Could you check a few things on this model? Use its own coordinates, in mm. A direction names the side the tool comes from. Give positions to 0.01 mm unless a question says otherwise; leave off trailing zeros. Loops run counter-clockwise (first coordinate to the right, second up) from the corner with the lowest first, then second, coordinate; pieces in that order, holes last.
1. For P1, Ø6, axis at x = 77.5, y = 2.5, coming from the -Z side; P2, Ø6.5, axis at x = 66.94, z = 2.99, coming from the +Y side; P3, Ø1, axis at x = -1.5, y = 5, coming from the -Z side, each with a flat end and sliding along its axis, tell me the tip position at first contact or that it passes through.
2. Imagine slicing it at C-C (x = -82.5). List the corners of the cut face in (y, z) for me.
3. Imagine slicing it at A-A (y = 10.25). Count the separate pieces of the cut face and the enclosed holes in it, plus the area to 3 significant figures.
4. For faces 1 (the cylindrical face through (100.424, 3.757, -33.251)), 2 (the flat face through (110, 7.62, -12)), which set-ups out of +Z, -Z, +X, -X, +Y, -Y let a thin tool reach every point of the face, with its end or its side?
5. I need wall thicknesses on line 1 along Z through (x, y) = (0, 8.5); line 2 along X through (y, z) = (10.25, 3); line 3 along Z through (x, y) = (45, 10.25). Which ranges of each line are inside material? Lowest first, please.
6. Thinking about a two-plate mould opening in Z: for faces 3 (the flat face through (86.8, 7.62, 8.5)), 4 (the flat face through (1, 6, 69.85)), 5 (the flat face through (29, 12.7, 19)), which applies, +Z half, -Z half, draft (parallel to the pull), parting line (faces both ways), or undercut?
7. Imagine slicing it at B-B (z = 22.5). List the corners of the cut face in (x, y) for me, plus the area to 3 significant figures.
```python
from build123d import *

# Parameters (mm, degrees)
SKETCH1_R                              = 14.2875
SKETCH1_R_2                            = 1.27
INITIAL_PLATE_DEPTH                    = 12.7
PLATE_FILLET_R                         = 12.7
F_10_0_1935_INITIAL_FRONT_BRACE_HOLE_D = 4.9149
SKETCH18_R                             = 2.65745
BOLT_CLEARANCE_DEPTH                   = 13.7
MOUNTING_PATTERN_COUNT                 = 18
MOUNTING_PATTERN_PITCH                 = 12.7
SKETCH21_R                             = 1.27
CHURRO_SUPPORT_PILOT_HOLE_DEPTH        = 13.7
F_1_4_0_25_DIAMETER_HOLE1_D            = 6.35
SKETCH25_R                             = 6.35
BOLT_HEAD_HOLE_DEPTH                   = 5.842
SKETCH12_R                             = 1.27
MAXPLANETARY_PILOT_HOLES_DEPTH         = 13.7
F_10_0_1935_MAXPLANETARY_MOUNTING_D    = 4.9149
SKETCH19_R                             = 2.65745
BOLT_HOLE_CLEARANCE_DEPTH              = 13.7
SKETCH12_3_R                           = 4.445
SKETCH12_3_R_2                         = 1.27
MAX_BOLT_HEAD_CLEARANCE_DEPTH          = 5.08
MAXPLANETARY_MOUNTING_PATTERN_COUNT    = 2
MAXPLANETARY_MOUNTING_PATTERN_ANGLE    = 90


with BuildPart() as part:
    # Sketch1 → Initial Plate (new body)
    with BuildSketch(Plane(origin=(0, 0, 0), x_dir=(1, 0, 0), z_dir=(0, 1, 0))):
        with BuildLine():
            Line((77.181752763, 58.744938329), (-7.718661497, 43.774704621))
            ThreePointArc((-7.718661497, 43.774704621), (-19.485598541, 39.951394838), (-29.742857216, 33.032785904))
            Line((-29.742857216, 33.032785904), (-144.005766802, -69.85))
            Line((-144.005766802, -69.85), (129.35041426, -69.85))
            Line((129.35041426, -69.85), (129.35041426, 59.420233707))
            Line((129.35041426, 59.420233707), (84.900414295, 59.420233707))
            ThreePointArc((84.900414295, 59.420233707), (81.026341512, 59.251088039), (77.181752763, 58.744938329))
        make_face()
        Circle(SKETCH1_R, mode=Mode.SUBTRACT)
        with Locations((84.90041426, 14.970233707)):
            Circle(SKETCH1_R, mode=Mode.SUBTRACT)
        with Locations((114.11041426, -57.15)):
            Circle(SKETCH1_R_2, mode=Mode.SUBTRACT)
    extrude(amount=INITIAL_PLATE_DEPTH)

    # Plate Fillet
    plate_fillet_edges = [part.edges().sort_by_distance(p)[0] for p in [
        (129.35041426, 6.35, 69.85),
        (-144.005766802, 6.35, 69.85),
        (129.35041426, 6.35, -59.420233707),
    ]]
    fillet(plate_fillet_edges, radius=PLATE_FILLET_R)

    # 10 _0.1935_ Initial Front Brace Hole (through all)
    with Locations(Plane(origin=(0, 12.7, 0), x_dir=(1, 0, 0), z_dir=(0, 1, 0))):
        with Locations((114.11041426, -57.15)):
            f_10_0_1935_initial_front_brace_hole = Hole(F_10_0_1935_INITIAL_FRONT_BRACE_HOLE_D / 2)

    # Sketch18 → Bolt Clearance (cut, through all)
    with BuildSketch(Plane(origin=(0, 12.7, 0), x_dir=(1, 0, 0), z_dir=(0, 1, 0))):
        with Locations((114.11041426, -57.15)):
            Circle(SKETCH18_R)
    extrude(amount=-BOLT_CLEARANCE_DEPTH, mode=Mode.SUBTRACT)

    # Mounting Pattern: 10 _0.1935_ Initial Front Brace Hole ×18
    with Locations(*[(-i * MOUNTING_PATTERN_PITCH, 0, 0) for i in range(1, MOUNTING_PATTERN_COUNT)]):
        add(f_10_0_1935_initial_front_brace_hole, mode=Mode.SUBTRACT)

    # Sketch21 → Churro Support Pilot Hole (cut, through all)
    with BuildSketch(Plane(origin=(0, 12.7, 0), x_dir=(1, 0, 0), z_dir=(0, 1, 0))):
        with Locations((116.65041426, 46.720233707)):
            Circle(SKETCH21_R)
    extrude(amount=-CHURRO_SUPPORT_PILOT_HOLE_DEPTH, mode=Mode.SUBTRACT)

    # 1_4 _0.25_ Diameter Hole1 (through all)
    with Locations(Plane(origin=(0, 12.7, 0), x_dir=(1, 0, 0), z_dir=(0, 1, 0))):
        with Locations((116.65041426, 46.720233707), (114.11041426, -57.15)):
            Hole(F_1_4_0_25_DIAMETER_HOLE1_D / 2)

    # Sketch25 → Bolt Head Hole (cut)
    with BuildSketch(Plane(origin=(0, 12.7, 0), x_dir=(1, 0, 0), z_dir=(0, 1, 0))):
        with Locations((116.65041426, 46.720233707)):
            Circle(SKETCH25_R)
    extrude(amount=-BOLT_HEAD_HOLE_DEPTH, mode=Mode.SUBTRACT)

    # Sketch12 → MaxPlanetary Pilot Holes (cut, through all)
    with BuildSketch(Plane(origin=(0, 12.7, 0), x_dir=(1, 0, 0), z_dir=(0, 1, 0))):
        with Locations((66.939902018, 32.93074595)):
            Circle(SKETCH12_R)
        with Locations((59.50041426, 14.970233707)):
            Circle(SKETCH12_R)
        with Locations((110.30041426, 14.970233707)):
            Circle(SKETCH12_R)
        with Locations((102.860926502, -2.990278535)):
            Circle(SKETCH12_R)
    extrude(amount=-MAXPLANETARY_PILOT_HOLES_DEPTH, mode=Mode.SUBTRACT)

    # 10 _0.1935_ MaxPlanetary Mounting (through all)
    with Locations(Plane(origin=(0, 12.7, 0), x_dir=(1, 0, 0), z_dir=(0, 1, 0))):
        with Locations((59.50041426, 14.970233707), (66.939902018, 32.93074595), (110.30041426, 14.970233707), (102.860926502, -2.990278535)):
            f_10_0_1935_maxplanetary_mounting = Hole(F_10_0_1935_MAXPLANETARY_MOUNTING_D / 2)

    # Sketch19 → Bolt Hole Clearance (cut, through all)
    with BuildSketch(Plane(origin=(0, 12.7, 0), x_dir=(1, 0, 0), z_dir=(0, 1, 0))):
        with Locations((66.939902018, 32.93074595)):
            Circle(SKETCH19_R)
        with Locations((59.50041426, 14.970233707)):
            Circle(SKETCH19_R)
        with Locations((110.30041426, 14.970233707)):
            Circle(SKETCH19_R)
        with Locations((102.860926502, -2.990278535)):
            Circle(SKETCH19_R)
    extrude(amount=-BOLT_HOLE_CLEARANCE_DEPTH, mode=Mode.SUBTRACT)

    # Sketch12_3 → Max Bolt Head Clearance (cut)
    with BuildSketch(Plane(origin=(0, 12.7, 0), x_dir=(1, 0, 0), z_dir=(0, 1, 0))):
        with Locations((66.939902018, 32.93074595)):
            Circle(SKETCH12_3_R)
        with Locations((66.939902018, 32.93074595)):
            Circle(SKETCH12_3_R_2, mode=Mode.SUBTRACT)
        with Locations((59.50041426, 14.970233707)):
            Circle(SKETCH12_3_R)
        with Locations((59.50041426, 14.970233707)):
            Circle(SKETCH12_3_R_2, mode=Mode.SUBTRACT)
        with Locations((102.860926502, -2.990278535)):
            Circle(SKETCH12_3_R)
        with Locations((102.860926502, -2.990278535)):
            Circle(SKETCH12_3_R_2, mode=Mode.SUBTRACT)
        with Locations((110.30041426, 14.970233707)):
            Circle(SKETCH12_3_R)
        with Locations((110.30041426, 14.970233707)):
            Circle(SKETCH12_3_R_2, mode=Mode.SUBTRACT)
    max_bolt_head_clearance = extrude(amount=-MAX_BOLT_HEAD_CLEARANCE_DEPTH, mode=Mode.SUBTRACT)

    # MaxPlanetary Mounting Pattern: 10 _0.1935_ MaxPlanetary Mounting, Max Bolt Head Clearance ×2 about axis
    maxplanetary_mounting_pattern_axis = Axis((84.90041426, 0, -14.970233707), (0, 1, 0))
    for i in range(1, MAXPLANETARY_MOUNTING_PATTERN_COUNT):
        add(f_10_0_1935_maxplanetary_mounting.rotate(maxplanetary_mounting_pattern_axis, i * MAXPLANETARY_MOUNTING_PATTERN_ANGLE / (MAXPLANETARY_MOUNTING_PATTERN_COUNT - 1)), mode=Mode.SUBTRACT)
        add(max_bolt_head_clearance.rotate(maxplanetary_mounting_pattern_axis, i * MAXPLANETARY_MOUNTING_PATTERN_ANGLE / (MAXPLANETARY_MOUNTING_PATTERN_COUNT - 1)), mode=Mode.SUBTRACT)


solid = part.part
```
Derived:
1. P1: stops at z = -59.2
1. P2: stops at y = 7.62
1. P3: stops at z = -44.96
2. outline: (0, 14.47) - (12.7, 14.47) - (12.7, 69.85) - (0, 69.85) - close
3. separate pieces: 1
3. enclosed holes: 29
3. area: 22,800 mm2
4. face 1: +Y, -Y
4. face 2: +Y
5. line 1: z = -45.14 to -14.29, 14.29 to 54.7, 59.6 to 69.85
5. line 2: x = -69.76 to -13.97, 13.97 to 62.49, 71.38 to 98.42, 107.31 to 129.35
5. line 3: z = -53.07 to 69.85
6. face 3: undercut
6. face 4: +Z half
6. face 5: draft
7. outline: (-91.42, 0) - (129.35, 0) - (129.35, 12.7) - (-91.42, 12.7) - close
7. area: 2,800 mm2
